Job drawing, mm, ordinate dimensions from the low corner. One solid piece. A direction names the side the tool comes from. Coordinates: 2 decimals unless noted, no trailing zeros. Loops run counter-clockwise (first coordinate to the right, second up) from the corner with the lowest first, then second, coordinate; pieces in that order, holes last. Notation, with made-up numbers: (55.25, 6.5) - (87.25, 6.5) arc R26 ccw to (87.25, 42.5) - close; hole circle Ø11 at (51, -27). An arc over 180 degrees is marked (long way). Use a Markdown table: item, result. Add a question column.
1. Band-saw the part on B-B, the plane y = 18.5. Give the cut face in (x, z).
2. Pull direction X, two halves, no side cores. Call the marked faces 3, 4, 5 and 6: pulls with the +X half, pulls with the -X half, needs draft (parallel to the pull), parting line crosses it, or undercut.
3. Drop a flat-ended pin along its axis: pin 1 (1 mm diameter, centred on x = 24, y = 31, fed in from -Z). Give the stop position or say it passes through.
4. Band-saw the part on A-A, the plane z = 0.9. Give the cut face in (x, y) (1 decimal).
5. Wall check: probe 1 along X at (y, z) = (17.5, 1.7); probe 2 along Y at (x, z) = (17.5, 2.65); probe 3 along X at (y, z) = (4, 0.8). Give the ranges that are in metal, low to high. Write a range as [from, to].
6. Band-saw the part on C-C, the plane x = 9. Give the cut face in (y, z), plus the area to 3 significant figures.
7. 3-axis set-ups, long thin cutter, end or side, ignore diameter. For the marked faces 1 and 2: which of +Z, -Z, +X, -X, +Y, -Y reach the whole face in a straight line?
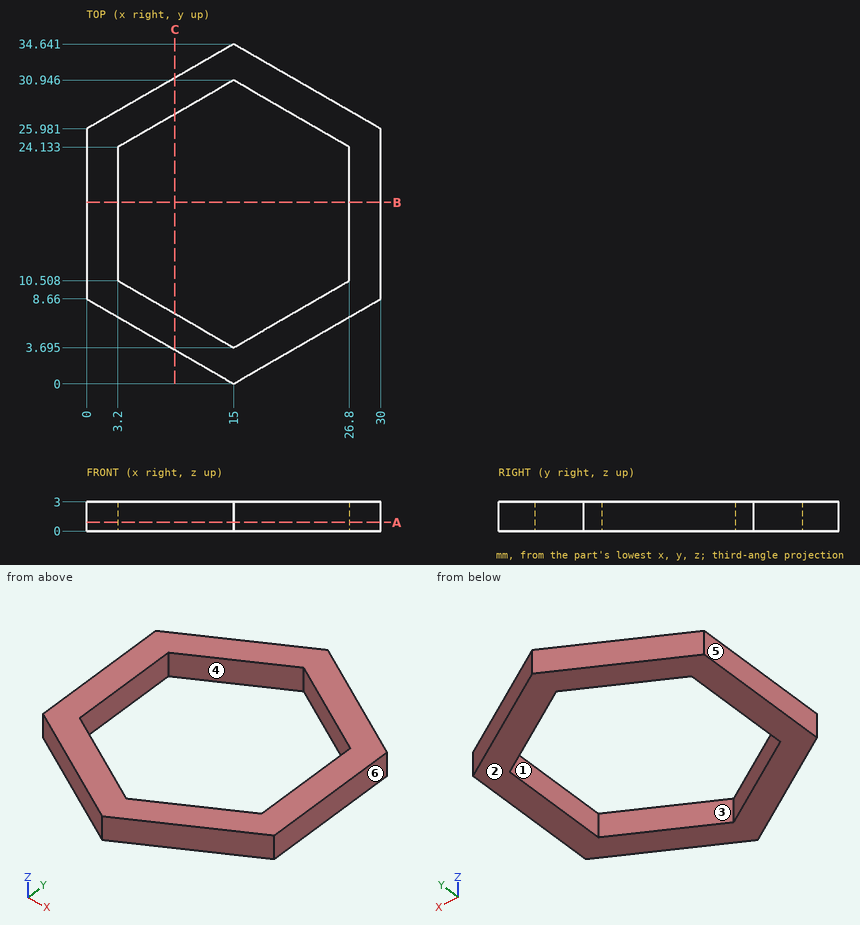
Geometry check:
| question | item | result |
|---|---|---|
| 1 | outline | (0, 0) - (3.2, 0) - (3.2, 3) - (0, 3) - close; (26.8, 0) - (30, 0) - (30, 3) - (26.8, 3) - close |
| 2 | face 3 | undercut |
| 2 | face 4 | undercut |
| 2 | face 5 | pulls with the -X half |
| 2 | face 6 | pulls with the +X half |
| 3 | pin 1 | passes through |
| 4 | outline | (0, 8.7) - (15, 0) - (30, 8.7) - (30, 26) - (15, 34.6) - (0, 26) - close; hole (3.2, 10.5) - (15, 3.7) - (26.8, 10.5) - (26.8, 24.1) - (15, 30.9) - (3.2, 24.1) - close |
| 5 | probe 1 | x = [0, 3.2], [26.8, 30] |
| 5 | probe 2 | y = [1.44, 5.14], [29.5, 33.2] |
| 5 | probe 3 | x = [8.07, 14.47], [15.53, 21.93] |
| 6 | outline | (3.46, 0) - (7.16, 0) - (7.16, 3) - (3.46, 3) - close; (27.48, 0) - (31.18, 0) - (31.18, 3) - (27.48, 3) - close |
| 6 | area | 22.2 mm^2 |
| 7 | face 1 | +Z, -Z |
| 7 | face 2 | -Z, +X, -X, +Y, -Y |
